from build123d import *

# Parameters (mm, degrees)
SKETCH1_W           = 99.999999898
SKETCH1_H           = 54.999999982
BOSS_EXTRUDE4_DEPTH = 5
BOSS_EXTRUDE6_DEPTH = 13
SKETCH2_3_W         = 5
SKETCH2_3_H         = 10
BOSS_EXTRUDE7_DEPTH = 3
SKETCH4_R           = 2
BOSS_EXTRUDE8_DEPTH = 8


with BuildPart() as part:
    # Sketch1 → Boss-Extrude4 (new body)
    with BuildSketch(Plane(origin=(0, 0, 0), x_dir=(1, 0, 0), z_dir=(0, 1, 0))):
        with Locations((31.542022725, 14.806957854)):
            Rectangle(SKETCH1_W, SKETCH1_H)
    extrude(amount=-BOSS_EXTRUDE4_DEPTH)

    # Sketch2 → Boss-Extrude6 (add)
    with BuildSketch(Plane(origin=(0, 0, 0), x_dir=(1, 0, 0), z_dir=(0, 1, 0))):
        Polygon((81.542022674, 42.306957845), (-18.457977224, 42.306957845), (-18.457977224, 17.306957845), (-13.457977224, 17.306957845), (-13.457977224, 37.306957845), (76.542022776, 37.306957845), (76.542022776, -7.693042155), (-13.457977224, -7.693042155), (-13.457977224, 7.306957845), (-18.457977224, 7.306957845), (-18.457977224, -12.693042137), (81.542022674, -12.693042137), align=None)
    extrude(amount=BOSS_EXTRUDE6_DEPTH)

    # Sketch2_3 → Boss-Extrude7 (add)
    with BuildSketch(Plane(origin=(0, 0, 0), x_dir=(1, 0, 0), z_dir=(0, 1, 0))):
        with Locations((-15.957977224, 12.306957845)):
            Rectangle(SKETCH2_3_W, SKETCH2_3_H)
    extrude(amount=BOSS_EXTRUDE7_DEPTH)

    # Sketch4 → Boss-Extrude8 (add)
    with BuildSketch(Plane(origin=(0, 0, 0), x_dir=(1, 0, 0), z_dir=(0, 1, 0))):
        with Locations(Location((-8.957977224, 32.806957845, 0), (0, 0, 270))):
            Circle(SKETCH4_R)
        with Locations(Location((-8.957977224, -3.193042155, 0), (0, 0, 270))):
            Circle(SKETCH4_R)
        with Locations(Location((71.542022776, -3.193042155, 0), (0, 0, 270))):
            Circle(SKETCH4_R)
        with Locations(Location((71.542022776, 32.306957845, 0), (0, 0, 270))):
            Circle(SKETCH4_R)
    extrude(amount=BOSS_EXTRUDE8_DEPTH)


solid = part.part
For this review, take the finished solid that the model builds, in its own axes (mm). A direction names the side the tool comes from. Coordinates: 2 decimals unless noted, no trailing zeros. Loops run counter-clockwise (first coordinate to the right, second up) from the corner with the lowest first, then second, coordinate; pieces in that order, holes last. Notation, with made-up numbers: (64.25, -7.5) -> (113.25, -7.5) arc R31 cw to (113.25, 16.5) -> close; hole circle Ø6 at (33, -0.5). An arc over 180 degrees is marked (long way). Write each question's results on one line, items separated by ' | '.
Q1. Mouldability with a two-part tool opening along Z and no side actions: class faces 1 (the flat face through (-9, 8, -33)), 2 (the flat face through (31, 4, 12.693)), 3 (the flat face through (-9, 8, 3)), 4 (the flat face through (81.542, 4, -14)) as +Z half, -Z half, draft (parallel to the pull), parting line (faces both ways), or undercut.
Taken from the geometry:
face 1: undercut | face 2: +Z half | face 3: undercut | face 4: draft
Q2. Machinability: for faces 5 (the flat face through (-16, 8, -17.307)), 6 (the flat face through (76.542, 6, -15)), 7 (the flat face through (31, 13, -39)), which of the approach directions +Z, -Z, +X, -X, +Y, -Y give a long, thin tool a straight path to every point of the face, cutting with its end or side? Answer none if there is none.
Taken from the geometry:
face 5: -X, +Y | face 6: +Y | face 7: +Z, -Z, +X, -X, +Y
Q3. Add section C-C, the plane y = 11.75. State the section outline as (x, z) points.
Taken from the geometry:
outline: (-18.46, -42.31) -> (81.54, -42.31) -> (81.54, 12.69) -> (-18.46, 12.69) -> (-18.46, -7.31) -> (-13.46, -7.31) -> (-13.46, 7.69) -> (76.54, 7.69) -> (76.54, -37.31) -> (-13.46, -37.31) -> (-13.46, -17.31) -> (-18.46, -17.31) -> close
Q4. To check wall thickness, follow line 1 along Z through (x, y) = (-12, 7.75); line 2 along X through (y, z) = (8.75, -26); line 3 along X through (y, z) = (4.25, -32). State the ranges of each line that lie inside material, in increasing order. Write a range as [from, to].
Taken from the geometry:
line 1: [-42.31, -37.31], [7.69, 12.69] | line 2: [-18.46, -13.46], [76.54, 81.54] | line 3: [-18.46, -13.46], [-10.79, -7.13], [69.57, 73.52], [76.54, 81.54]
Q5. For pin 1 Ø3 at (x, z) = (71, -31.5) entering from +Y; pin 2 Ø8 at (x, z) = (55, -22.5) entering from +Y; pin 3 Ø4 at (y, z) = (9.5, -12) entering from -X, all flat-tipped, find the tip position at first contact; note any pin that passes through.
Taken from the geometry:
pin 1: y = 8 | pin 2: y = 0 | pin 3: x = 76.54
Q6. Add section B-B, the plane x = 65.5. State the section outline as (y, z) points.
Taken from the geometry:
outline: (-5, -42.31) -> (13, -42.31) -> (13, -37.31) -> (0, -37.31) -> (0, 7.69) -> (13, 7.69) -> (13, 12.69) -> (-5, 12.69) -> close
Q7. Add section A-A, the plane z = -18.5. State the section outline as (x, y) points.
Taken from the geometry:
outline: (-18.46, -5) -> (81.54, -5) -> (81.54, 13) -> (76.54, 13) -> (76.54, 0) -> (-13.46, 0) -> (-13.46, 13) -> (-18.46, 13) -> close
